```python
from build123d import *

# Parameters (mm, degrees)
SKETCH_1_W          = 36.75
SKETCH_1_H          = 21.4
SKETCH_1_R          = 1.5
EXTRUDE_1_DEPTH     = 10
SKETCH_1_16_R       = 2.25
CUT_EXTRUDE_1_DEPTH = 7
SKETCH_2_R          = 1
CUT_EXTRUDE_2_DEPTH = 2
CUT_EXTRUDE_START   = -19.4
SKETCH_2_2_R        = 1
CUT_EXTRUDE_3_DEPTH = 2
SKETCH_3_R          = 1
CUT_EXTRUDE_4_DEPTH = 4


with BuildPart() as part:
    # 草图1 → 凸台-拉伸1 (new body)
    with BuildSketch(Plane(origin=(0, 0, 0), x_dir=(1, 0, 0), z_dir=(0, 1, 0))):
        with Locations((-2, -3.2)):
            Rectangle(SKETCH_1_W, SKETCH_1_H)
        with Locations(Location((-8.375, 0, 0), (0, 0, 270))):
            Circle(SKETCH_1_R, mode=Mode.SUBTRACT)
        with BuildLine():
            ThreePointArc((5.5, 0), (0, -5.5), (-5.5, 0))
            ThreePointArc((-5.5, 0), (0, 5.5), (5.5, 0))
        make_face(mode=Mode.SUBTRACT)
        with Locations(Location((8.375, 0, 0), (0, 0, 270))):
            Circle(SKETCH_1_R, mode=Mode.SUBTRACT)
        with Locations(Location((0, -10.9, 0), (0, 0, 270))):
            Circle(SKETCH_1_R, mode=Mode.SUBTRACT)
    extrude(amount=EXTRUDE_1_DEPTH)

    # 草图1<16> → 切除-拉伸1 (cut)
    with BuildSketch(Plane(origin=(0, 0, 0), x_dir=(1, 0, 0), z_dir=(0, 1, 0))):
        with Locations(Location((-8.375, 0, 0), (0, 0, 270))):
            Circle(SKETCH_1_16_R)
        with Locations(Location((8.375, 0, 0), (0, 0, 270))):
            Circle(SKETCH_1_16_R)
        with Locations(Location((0, -10.9, 0), (0, 0, 270))):
            Circle(SKETCH_1_16_R)
    extrude(amount=CUT_EXTRUDE_1_DEPTH, mode=Mode.SUBTRACT)

    # 草图2 → 切除-拉伸2 (cut)
    with BuildSketch(Plane(origin=(0, 0, -7.5), x_dir=(-1, 0, 0), z_dir=(0, 0, -1))):
        with Locations((-11.375, 5)):
            Circle(SKETCH_2_R)
        with Locations((10.375, 5)):
            Circle(SKETCH_2_R)
    extrude(amount=-CUT_EXTRUDE_2_DEPTH, mode=Mode.SUBTRACT)

    # 草图2<2> → 切除-拉伸3 (cut)
    with BuildSketch(Plane(origin=(0, 0, -7.5), x_dir=(-1, 0, 0), z_dir=(0, 0, -1)).offset(CUT_EXTRUDE_START)):
        with Locations((-11.375, 5)):
            Circle(SKETCH_2_2_R)
        with Locations((10.375, 5)):
            Circle(SKETCH_2_2_R)
    extrude(amount=-CUT_EXTRUDE_3_DEPTH, mode=Mode.SUBTRACT)

    # 草图3 → 切除-拉伸4 (cut)
    with BuildSketch(Plane(origin=(16.375, 0, 0), x_dir=(0, 0, -1), z_dir=(1, 0, 0))):
        with Locations((-8.9, 5)):
            Circle(SKETCH_3_R)
        with Locations((3.5, 5)):
            Circle(SKETCH_3_R)
    extrude(amount=-CUT_EXTRUDE_4_DEPTH, mode=Mode.SUBTRACT)


solid = part.part
```
Build history of the part. All positions in model axes, mm. A direction names the side the tool comes from. Coordinates: 2 decimals unless noted, no trailing zeros. Order: outer loops, then holes, each group sorted by start corner. A loop starts at its lowest first (then second) coordinate and runs counter-clockwise, first axis right, second up.
Item 1: Saw through at C-C on x = 4.5. List the corners of the cut face in (y, z), then the cut area to 3 significant figures.
Filled in:
outline: (0, -7.5) - (10, -7.5) - (10, -3.16) - (0, -3.16) - close; (0, 3.16) - (10, 3.16) - (10, 13.9) - (0, 13.9) - close
area: 151 mm2
Item 2: Saw through at D-D on x = 0. List the corners of the cut face in (y, z), then the cut area to 3 significant figures.
Filled in:
outline: (0, -7.5) - (10, -7.5) - (10, -5.5) - (0, -5.5) - close; (0, 5.5) - (10, 5.5) - (10, 9.4) - (7, 9.4) - (7, 8.65) - (0, 8.65) - close; (0, 13.15) - (7, 13.15) - (7, 12.4) - (10, 12.4) - (10, 13.9) - (0, 13.9) - close
area: 63.5 mm2
Item 3: Saw through at A-A on z = 10.9. List the corners of the cut face in (x, y) (3 decimals).
Filled in:
outline: (-20.375, 0) - (-2.25, 0) - (-2.25, 7) - (-1.5, 7) - (-1.5, 10) - (-20.375, 10) - close; (1.5, 7) - (2.25, 7) - (2.25, 0) - (16.375, 0) - (16.375, 10) - (1.5, 10) - close
Item 4: Drill centre lines: L1, parallel to X at y = 2.5, z = 10.9 (3 decimals); L2, parallel to X at y = 1.5, z = -1 (3 decimals); L3, parallel to Z at x = -1, y = 9.5. Where is each one in solid material? Low to high.
Filled in:
L1: x = -20.375 to -2.25, 2.25 to 16.375
L2: x = -20.375 to -10.391, -6.359 to -5.408, 5.408 to 6.359, 10.391 to 16.375
L3: z = -7.5 to -5.41, 5.41 to 9.78, 12.02 to 13.9
Item 5: Drop flat-ended pins along their axis: pin 1 Ø1.6 at (y, z) = (5, -3.5) entering from +X (3 decimals); pin 2 Ø1 at (x, y) = (-10.5, 5) entering from +Z; pin 3 Ø1.2 at (x, y) = (-10.375, 5) entering from -Z; pin 4 Ø1 at (x, z) = (1.5, 4.5) entering from +Y. Give the stop position or say it passes through.
Filled in:
pin 1: stops at x = 12.375
pin 2: stops at z = 11.9
pin 3: stops at z = -5.5
pin 4: passes through
Item 6: Mould opens along Y. For faces 6 (the flat face through (11, 5, 11.9)), 7 (the flat face through (-2, 5, 13.9)), 8 (the flat face through (-2.3, 0, 5.4)) say: released by +Y, released by -Y, zero draft, split by the parting line, or undercut.
Filled in:
face 6: undercut
face 7: zero draft
face 8: released by -Y
Item 7: Tool access for faces 1 (the flat face through (7, 7, -1)), 2 (the cylindrical face through (14.4, 5.84, 8.36)), 3 (the cylindrical face through (12.11, 5.68, 12.89)), 4 (the cylindrical face through (0.07, 8.48, 9.4)), 5 (the cylindrical face through (12.11, 5.68, -6.51)): list every direction of +Z, -Z, +X, -X, +Y, -Y with a clear straight run to the whole face (end or side of a thin tool).
Filled in:
face 1: -Y
face 2: +X
face 3: +Z
face 4: +Y, -Y
face 5: -Z
Item 8: Saw through at B-B on z = 0. List the corners of the cut face in (x, y) (3 decimals).
Filled in:
outline: (-20.375, 0) - (-10.625, 0) - (-10.625, 7) - (-9.875, 7) - (-9.875, 10) - (-20.375, 10) - close; (-6.875, 7) - (-6.125, 7) - (-6.125, 0) - (-5.5, 0) - (-5.5, 10) - (-6.875, 10) - close; (5.5, 0) - (6.125, 0) - (6.125, 7) - (6.875, 7) - (6.875, 10) - (5.5, 10) - close; (9.875, 7) - (10.625, 7) - (10.625, 0) - (16.375, 0) - (16.375, 10) - (9.875, 10) - close
